```python
from build123d import *

# Parameters (mm, degrees)
PAD_DEPTH     = 51.5
THICKNESS_T   = -0.5
SKETCH002_W   = 5
SKETCH002_H   = 12
SKETCH002_W_2 = 2
SKETCH002_H_2 = 8
POCKET_DEPTH  = 5


with BuildPart() as part:
    # Sketch → Pad (new body, symmetric)
    with BuildSketch(Plane.XZ):
        with BuildLine():
            Line((16.5, -4.48614), (16.5, 1.35978))
            add(Edge.make_bspline(
                [(10.5, 6.5), (14.0348, 4.18709), (16.5, 1.35978)],
                knots=[0, 0, 0, 1, 1, 1], degree=2))
            Line((10.5, 6.5), (-14.47, 2))
            Line((-14.47, 2), (-16.5, 0.15))
            Line((-16.5, 0.15), (-16.5, -4.65))
            Line((-16.5, -4.65), (-14.466996, -6.5))
            Line((-14.466996, -6.5), (10.5, -6.5))
            add(Edge.make_bspline(
                [(16.5, -4.48614), (13.35, -5.95741), (10.5, -6.5)],
                knots=[0, 0, 0, 1, 1, 1], degree=2))
        make_face()
    extrude(amount=PAD_DEPTH, both=True)

    # Thickness
    thickness_openings = [part.faces().sort_by_distance(p)[0] for p in [
        (0.779746, 51.5, -1.023703),
    ]]
    offset(amount=THICKNESS_T, openings=thickness_openings, kind=Kind.INTERSECTION)

    # Sketch002 (on Face1 of Pad) → Pocket (cut)
    with BuildSketch(Plane(origin=(16.5, 0, 0), x_dir=(0, 0, 1), z_dir=(1, 0, 0))):
        with Locations((-1.56114, 9.5)):
            Rectangle(SKETCH002_W, SKETCH002_H)
        with Locations((-1.56114, -28.5)):
            Rectangle(SKETCH002_W, SKETCH002_H)
        with Locations((-1.56114, -9.5)):
            Rectangle(SKETCH002_W, SKETCH002_H)
        with Locations((-1.56022, 33.370129)):
            Rectangle(SKETCH002_W_2, SKETCH002_H_2)
    extrude(amount=-POCKET_DEPTH, mode=Mode.SUBTRACT)


solid = part.part
```
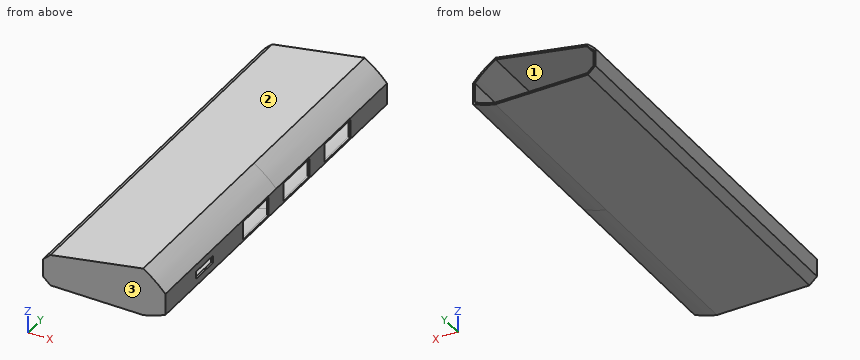
Could you check a few things on this model? Use its own coordinates, in mm. Face numbers are marked on the shaded views. Coordinates: 2 decimals unless noted, no trailing zeros. Loops run counter-clockwise (first coordinate to the right, second up) from the corner with the lowest first, then second, coordinate; pieces in that order, holes last. Notation, with made-up numbers: M -3.75,-11 L 12.25,-11 A23 ccw 12.25,19 Z; hole C 20.5,7 d8. An arc over 180 degrees is marked long. Put each result on its own line as item: value. Start each with the question number.
(1) Thinking about a two-plate mould opening in Z: for the marked faces 1, 2 and 3, which applies, pulls with the +Z half, pulls with the -Z half, needs draft (parallel to the pull), parting line crosses it, or undercut?
(2) I need wall thicknesses on line 1 (X direction, y = 38, z = -1); line 2 (Y direction, x = 9.5, z = -4.5); line 3 (Z direction, x = -2.5, y = 47). Which ranges of each line are inside material? Lowest first, please. Write a range as from..to.
(3) Suppose I cut it at A-A on x = -4.5. Please give me the cut outline in (y, z), then the cut area to 3 significant figures.
(4) Will these pins go through, and if not, where does the flat tip stop? P1, Ø6, axis at x = 5.5, y = 35, coming from the +Z side; P2, Ø0.6, axis at x = 16, y = 10, coming from the +Z side; P3, Ø3, axis at x = 1.5, z = -1, coming from the +Y side.
Solutions:
1. face 1: undercut
1. face 2: pulls with the +Z half
1. face 3: needs draft
2. line 1: x = -16.5..-16, 16..16.5
2. line 2: y = -51.5..-51
2. line 3: z = -6.5..-6, 3.65..4.16
3. outline: M -51.5,-6.5 L 51.5,-6.5 L 51.5,-6 L -51,-6 L -51,3.29 L 51.5,3.29 L 51.5,3.8 L -51.5,3.8 Z
3. area: 108 mm2
4. P1: stops at z = 6.14
4. P2: stops at z = 2.23
4. P3: stops at y = -51
